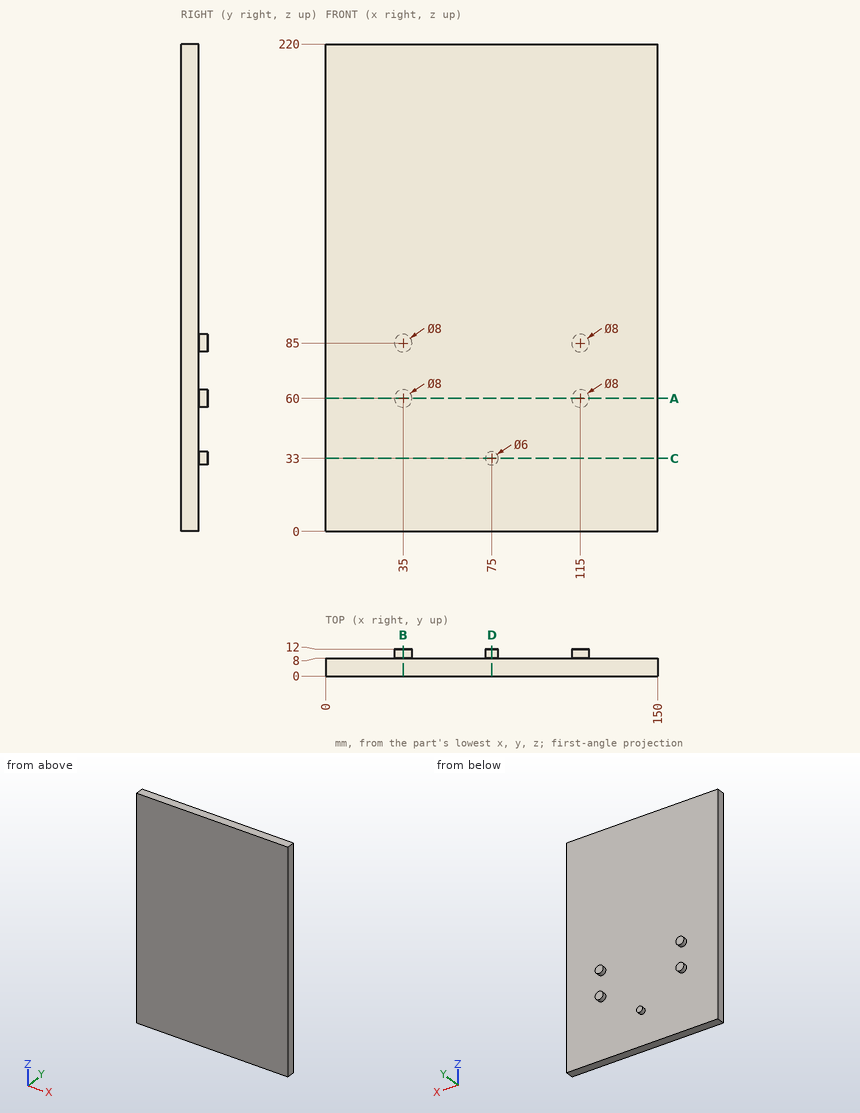
Source: three-view drawing plus pictorial views. Frame: mm from the lowest corner of the part. Round coordinates to 2 decimals unless told otherwise and drop trailing zeros. Loops run counter-clockwise (first coordinate to the right, second up) from the corner with the lowest first, then second, coordinate; pieces in that order, holes last.
Q1. Section C-C, the plane z = 33. Return loops of the section in (x, y).
Q2. First-contact query: P1, Ø2, axis at x = 51, z = 176, coming from the +Y side. Flat tip, straight axial feed; report the tip coordinate or a pass-through.
Q3. Section D-D, the plane x = 75. Return loops of the section in (y, z), plus the area to 3 significant figures.
Q4. Section A-A, the plane z = 60. Return loops of the section in (x, y).
Q5. Ray query, line 1 (Y direction, x = 57.5, z = 133); line 2 (Z direction, x = 38.5, y = 11.75); line 3 (Z direction, x = 77, y = 8.25). Return the intervals inside material, ascending.
Q6. Section B-B, the plane x = 35. Return loops of the section in (y, z), plus the area to 3 significant figures.
Solutions:
1. outline: (0, 0) - (150, 0) - (150, 8) - (78, 8) - (78, 12) - (72, 12) - (72, 8) - (0, 8) - close
2. P1: stops at y = 8
3. outline: (0, 0) - (8, 0) - (8, 30) - (12, 30) - (12, 36) - (8, 36) - (8, 220) - (0, 220) - close
3. area: 1,780 mm2
4. outline: (0, 0) - (150, 0) - (150, 8) - (119, 8) - (119, 12) - (111, 12) - (111, 8) - (39, 8) - (39, 12) - (31, 12) - (31, 8) - (0, 8) - close
5. line 1: y = 0 to 8
5. line 2: z = 58.06 to 61.94, 83.06 to 86.94
5. line 3: z = 30.76 to 35.24
6. outline: (0, 0) - (8, 0) - (8, 56) - (12, 56) - (12, 64) - (8, 64) - (8, 81) - (12, 81) - (12, 89) - (8, 89) - (8, 220) - (0, 220) - close
6. area: 1,820 mm2
